The listing builds one solid part. Answer for the finished solid, in the listing's coordinates (mm). A direction names the side the tool comes from. Coordinates: 2 decimals unless noted, no trailing zeros. Order: outer loops, then holes, each group sorted by start corner. A loop starts at its lowest first (then second) coordinate and runs counter-clockwise, first axis right, second up. Notation, with made-up numbers: (-38, -34) -> (-10, -34) arc R24 cw to (-10, -7) -> close; hole circle Ø8 at (40.25, -2.75). An arc over 180 degrees is marked (long way). Write each question's results on one line, items separated by ' | '. Start each with the question number.
(1) The part is cut by section B-B, the plane x = 70. Give the vertices of the cut face in (y, z).
(2) Determine the mould class of faces 5 (the face through (0, 28, -1)), 6 (the face through (56, 55, -1)), 7 (the face through (65, 28, -3)) for opening direction X: +X half, -X half, draft (parallel to the pull), parting line (faces both ways), or undercut.
(3) Straight lines are drawn through the part: L1, parallel to Y at x = 75, z = -4; L2, parallel to Y at x = 105, z = -2; L3, parallel to X at y = 14.5, z = -2.5. For each, find the intervals that lie inside material, in ascending order.
(4) A tool of negligible diameter and unlimited length cuts with its end or side. For faces 1 (the face through (9, 30, -1)), 2 (the face through (54, 48, -4)), 3 (the face through (56, 7, -4)), 4 (the face through (12.84, 14.24, -6.23)), from which of +Z, -Z, +X, -X, +Y, -Y can it reach the whole face along a straight path? Write none if from no direction.
(5) Given pin 1 (2 mm diameter, centred on x = 12.5, z = -6.5, fed in from +Y); pin 2 (20.5 mm diameter, centred on x = 32, y = 24, fed in from -Z); pin 3 (1.5 mm diameter, centred on y = 28, z = -4, fed in from -X), each flat-ended and moving along its own axis, determine where each tip first touches the part or whether it passes through.
(6) The part is cut by section C-C, the plane x = 30. Give the vertices of the cut face in (y, z), then the cut area to 3 significant figures.
(7) The part is cut by section A-A, the plane y = 28. Give the vertices of the cut face in (x, z).
(8) The part is cut by section D-D, the plane y = 37.5. Give the vertices of the cut face in (x, z).
Autodesk Fusion 360 part; units mm, degrees
sketch "Sketch2" plane through (0, 0, 0) normal (0, 0, 1) x (1, 0, 0)
  line L0 (5, 0) -> (105, 0)
  line L1 (110, 5) -> (110, 50)
  line L2 (105, 55) -> (5, 55)
  line L3 (0, 50) -> (0, 5)
  line L4 (10, 45) -> (45, 45)
  line L5 (45, 45) -> (45, 10)
  line L6 (45, 10) -> (10, 10)
  line L7 (10, 10) -> (10, 45)
  circle A0 centre (95, 40) radius 3.75
  circle A1 centre (70, 40) radius 3.75
  circle A2 centre (95, 15) radius 2.5
  circle A3 centre (70, 15) radius 2.5
  line L8 (10, 39) -> (45, 39)
  line L9 (45, 39) -> (45, 20)
  line L10 (45, 20) -> (10, 20)
  line L11 (10, 20) -> (10, 39)
  circle A4 centre (13, 42) radius 1.25
  circle A5 centre (42, 42) radius 1.25
  circle A6 centre (13, 13) radius 1.25
  circle A7 centre (42, 13) radius 1.25
  circle A8 centre (13, 42) radius 2
  circle A9 centre (42, 42) radius 2
  circle A10 centre (13, 13) radius 2
  circle A11 centre (42, 13) radius 2
  circle A12 centre (5, 50) radius 2
  circle A13 centre (105, 50) radius 2
  circle A14 centre (5, 5) radius 2
  circle A15 centre (105, 5) radius 2
  arc A16 (5, 55) -> (0, 50) centre (5, 50) ccw
  arc A17 (110, 50) -> (105, 55) centre (105, 50) ccw
  arc A18 (105, 0) -> (110, 5) centre (105, 5) ccw
  arc A19 (0, 5) -> (5, 0) centre (5, 5) ccw
  line L12 (8, 47) -> (102, 47)
  line L13 (102, 47) -> (102, 8)
  line L14 (102, 8) -> (8, 8)
  line L15 (8, 8) -> (8, 47)
  line L16 (7, 48) -> (103, 48)
  line L17 (103, 48) -> (103, 7)
  line L18 (103, 7) -> (7, 7)
  line L19 (7, 7) -> (7, 48)
  dimension "d3" = 7.5
  dimension "d4" = 20
  dimension "d5" = 10
  dimension "d6" = -25
  dimension "d7" = -25
  dimension "d8" = 5
  dimension "d9" = 20
  dimension "d10" = 10
  dimension "d11" = -25
  dimension "d12" = 0
  dimension "d13" = 2.5
  dimension "d14" = 20
  dimension "d15" = 20
  dimension "d16" = 29
  dimension "d17" = -29
  dimension "d18" = 4
  dimension "d19" = 20
  dimension "d20" = 20
  dimension "d21" = 29
  dimension "d22" = -29
  dimension "d23" = 4
  dimension "d24" = 20
  dimension "d25" = 20
  dimension "d26" = 100
  dimension "d27" = -45
  dimension "d28" = 5
extrude "Extrude1" add sketch "Sketch2" against normal blind 3 contours L0 L1 L2 L3 A16 A17 A18 A19 | L4 L5 L7 L8 | L5 L6 L7 L10 | L12 L13 L14 L15 makes body 1 at (71.066, 1.3774, 0) makes body 2 at (60.2764, 24.5895, 0)
extrude "Extrude2" add sketch "Sketch2" against normal blind 6 contours L16 L17 L18 L19 bodies 1 2
extrude "Extrude3" add sketch "Sketch2" against normal blind 4.5 contours A8 | A9 | A10 | A11 bodies 1
extrude "Extrude4" add sketch "Sketch2" against normal blind 8 contours A4 | A5 | A6 | A7 bodies 1
chamfer "Chamfer1" distance 2 angle 45 4 edges at (27.5, 20, 0) (27.5, 39, 0) (45, 29.5, 0) (10, 29.5, 0) on bodies 1
Established:
1) outline: (0, -3) -> (7, -3) -> (7, -6) -> (8, -6) -> (8, -3) -> (12.5, -3) -> (12.5, 0) -> (0, 0) -> close; (17.5, -3) -> (36.25, -3) -> (36.25, 0) -> (17.5, 0) -> close; (43.75, -3) -> (47, -3) -> (47, -6) -> (48, -6) -> (48, -3) -> (55, -3) -> (55, 0) -> (43.75, 0) -> close
2) face 5: -X half | face 6: draft | face 7: undercut
3) L1: y = 7 to 8, 47 to 48 | L2: y = 0 to 3, 7 to 48, 52 to 55 | L3: x = 0 to 67.55, 72.45 to 92.55, 97.45 to 110
4) face 1: +Z | face 2: -Z, +X, -X, +Y | face 3: -Z, +X, -X, -Y | face 4: -Z
5) pin 1: stops at y = 48 | pin 2: stops at z = -3 | pin 3: stops at x = 7
6) outline: (0, -3) -> (7, -3) -> (7, -6) -> (8, -6) -> (8, -3) -> (20, -3) -> (20, -2) -> (18, 0) -> (0, 0) -> close; (39, -3) -> (47, -3) -> (47, -6) -> (48, -6) -> (48, -3) -> (55, -3) -> (55, 0) -> (41, 0) -> (39, -2) -> close | area: 110 mm^2
7) outline: (0, -3) -> (7, -3) -> (7, -6) -> (8, -6) -> (8, -3) -> (10, -3) -> (10, -2) -> (8, 0) -> (0, 0) -> close; (45, -3) -> (102, -3) -> (102, -6) -> (103, -6) -> (103, -3) -> (110, -3) -> (110, 0) -> (47, 0) -> (45, -2) -> close
8) outline: (0, -3) -> (7, -3) -> (7, -6) -> (8, -6) -> (8, -3) -> (10, -3) -> (10, -2) -> (8, 0) -> (0, 0) -> close; (45, -3) -> (67.2, -3) -> (67.2, 0) -> (47, 0) -> (45, -2) -> close; (72.8, -3) -> (92.2, -3) -> (92.2, 0) -> (72.8, 0) -> close; (97.8, -3) -> (102, -3) -> (102, -6) -> (103, -6) -> (103, -3) -> (110, -3) -> (110, 0) -> (97.8, 0) -> close
